Could you check a few things on this drawing? It's one solid part, dimensions in mm from its lowest x, y, z. Round coordinates to 2 decimals unless told otherwise and drop trailing zeros. Write each loop counter-clockwise with the first axis right and the second up, starting at its lowest first coordinate (ties: lowest second). Pieces come first, ordered by that corner, then holes. Notation, with made-up numbers: (-35.75, 67.25) -> (5.25, 67.25) arc R37 cw to (5.25, 105.25) -> close; hole circle Ø4 at (47.25, 29). An arc over 180 degrees is marked (long way). Answer in a Markdown table with one row per item.
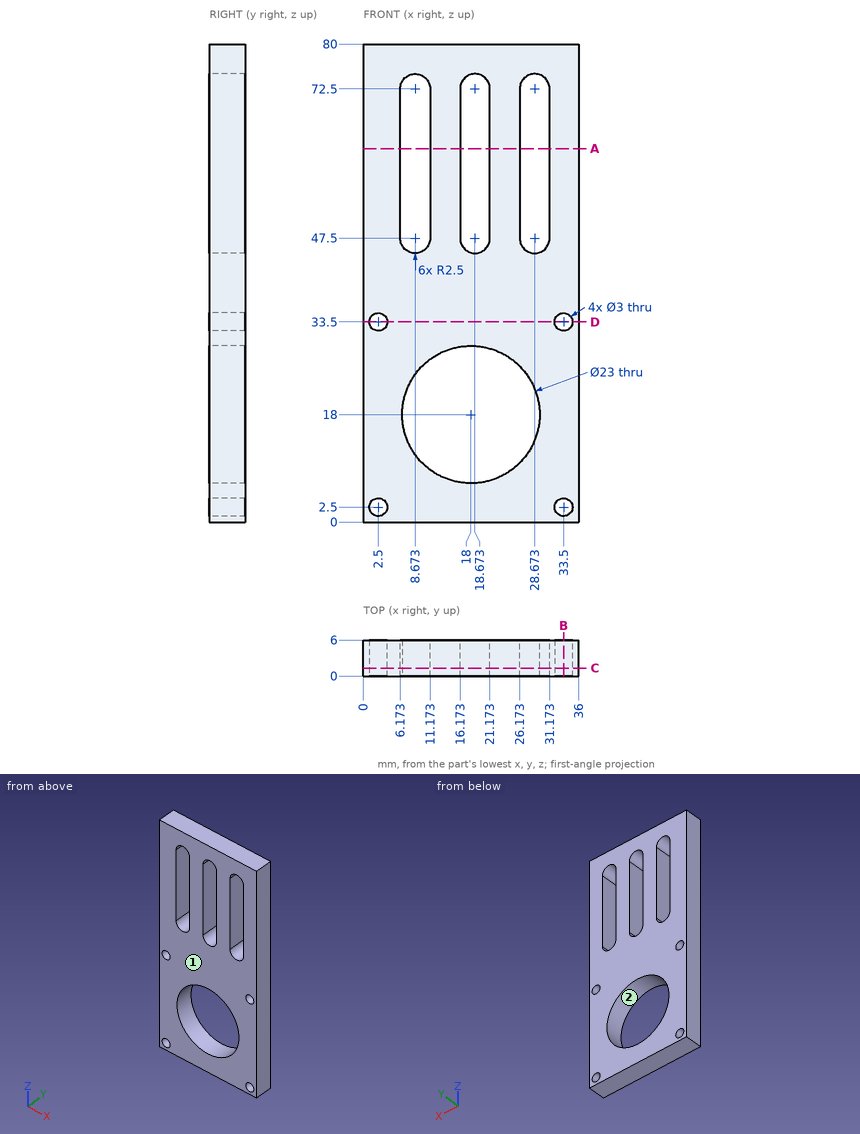
1) Imagine slicing it at A-A, the plane z = 62.5. Please give me the cut outline in (x, y), plus the area to 3 significant figures.
Findings:
| item | result |
|---|---|
| outline | (0, 0) -> (6.17, 0) -> (6.17, 6) -> (0, 6) -> close; (11.17, 0) -> (16.17, 0) -> (16.17, 6) -> (11.17, 6) -> close; (21.17, 0) -> (26.17, 0) -> (26.17, 6) -> (21.17, 6) -> close; (31.17, 0) -> (36, 0) -> (36, 6) -> (31.17, 6) -> close |
| area | 126 mm^2 |
2) Please list where these lines run through material, in increasing order: line 1 (X direction, y = 4.4, z = 33.5); line 2 (X direction, y = 1.75, z = 57); line 3 (Z direction, x = 33.5, y = 3.3).
Findings:
| item | result |
|---|---|
| line 1 | x = 0 to 1, 4 to 32, 35 to 36 |
| line 2 | x = 0 to 6.17, 11.17 to 16.17, 21.17 to 26.17, 31.17 to 36 |
| line 3 | z = 0 to 1, 4 to 32, 35 to 80 |
3) Imagine slicing it at B-B, the plane x = 33.5. Please give me the cut outline in (y, z).
Findings:
| item | result |
|---|---|
| outline | (0, 0) -> (6, 0) -> (6, 1) -> (0, 1) -> close; (0, 4) -> (6, 4) -> (6, 32) -> (0, 32) -> close; (0, 35) -> (6, 35) -> (6, 80) -> (0, 80) -> close |
4) Imagine slicing it at D-D, the plane z = 33.5. Please give me the cut outline in (x, y), plus the area to 3 significant figures.
Findings:
| item | result |
|---|---|
| outline | (0, 0) -> (1, 0) -> (1, 6) -> (0, 6) -> close; (4, 0) -> (32, 0) -> (32, 6) -> (4, 6) -> close; (35, 0) -> (36, 0) -> (36, 6) -> (35, 6) -> close |
| area | 180 mm^2 |
5) Imagine slicing it at C-C, the plane y = 1.3. Count the separate pieces of the cut face and the enclosed holes in it, plus the area to 3 significant figures.
Findings:
| item | result |
|---|---|
| separate pieces | 1 |
| enclosed holes | 8 |
| area | 2,000 mm^2 |
6) Thinking about a two-plate mould opening in Z: for the marked faces 1 and 2, which applies, +Z half, -Z half, draft (parallel to the pull), parting line (faces both ways), or undercut?
Findings:
| item | result |
|---|---|
| face 1 | draft |
| face 2 | undercut |
7) For pin 1 (2.5 mm diameter, centred on x = 33.5, z = 33.5, fed in from +Y), with a flat end and sliding along its axis, tell me the tip position at first contact or that it passes through.
Findings:
| item | result |
|---|---|
| pin 1 | passes through |
